Print and shaded views of the part. All mm, measured from the part's lowest x, y and z. A direction names the side the tool comes from. Give positions to 0.01 mm unless a question says otherwise; leave off trailing zeros. Write each loop counter-clockwise with the first axis right and the second up, starting at its lowest first coordinate (ties: lowest second). Pieces come first, ordered by that corner, then holes.
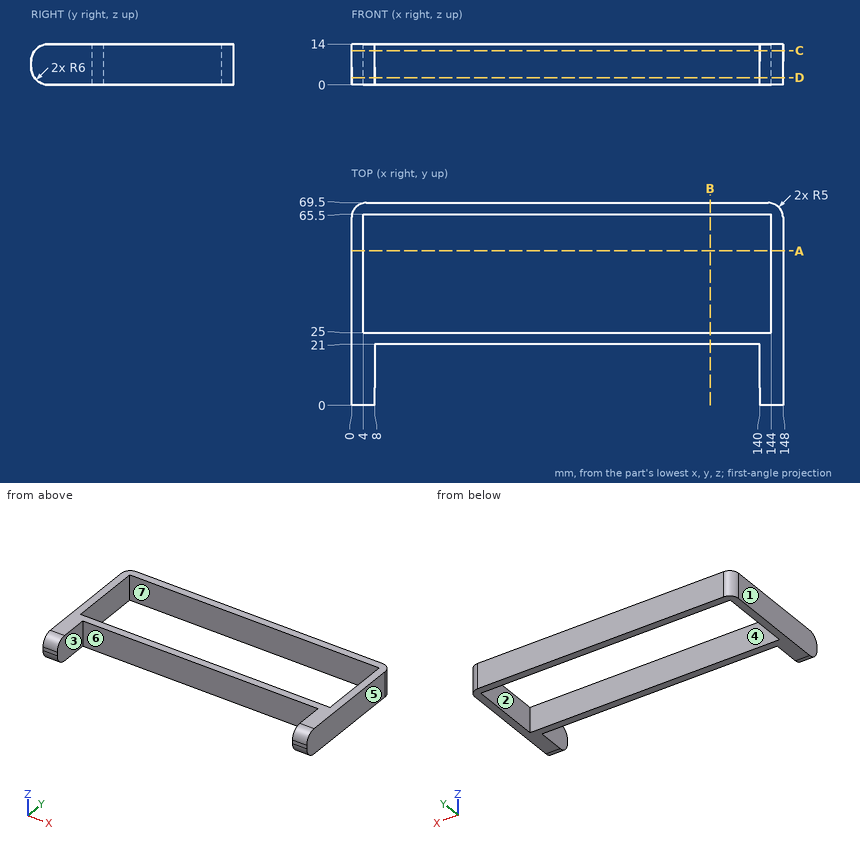
1. Saw through at C-C on z = 11.75. Give the cut face in (x, y), plus the area to 3 significant figures.
2. 3-axis set-ups, long thin cutter, end or side, ignore diameter. For the marked faces 1, 2 and 3: which of +Z, -Z, +X, -X, +Y, -Y reach the whole face in a straight line?
3. Saw through at D-D on z = 2.5. Give the cut face in (x, y), plus the area to 3 significant figures.
4. Saw through at A-A on y = 53. Give the cut face in (x, z), plus the area to 3 significant figures.
5. Drill centre lines: line 1 along Y through (x, z) = (42.5, 13); line 2 along X through (y, z) = (37, 8.75); line 3 along X through (y, z) = (15, 3.25). Where is each one in solid material? Low to high.
6. Mould opens along Y. For the marked faces 4, 5, 6 and 7 say: pulls with the +Y half, pulls with the -Y half, needs draft (parallel to the pull), parting line crosses it, or undercut.
7. Saw through at B-B on x = 123. Give the cut face in (y, z), plus the area to 3 significant figures.
8. Drop a flat-ended pin along its axis: pin 1 (3 mm diameter, centred on x = 132.5, z = 6, fed in from -Y). Give the stop position or say it passes through.
Outcome:
1. outline: (0, 1.32) - (8, 1.32) - (8, 21) - (140, 21) - (140, 1.32) - (148, 1.32) - (148, 64.5) arc R5 ccw to (143, 69.5) - (5, 69.5) arc R5 ccw to (0, 64.5) - close; hole (4, 25) - (144, 25) - (144, 65.5) - (4, 65.5) - close
1. area: 1,810 mm2
2. face 1: +Z, -Z, -X, +Y, -Y
2. face 2: +Z, -Z
2. face 3: +Z, -Z, -Y
3. outline: (0, 1.13) - (8, 1.13) - (8, 21) - (140, 21) - (140, 1.13) - (148, 1.13) - (148, 64.5) arc R5 ccw to (143, 69.5) - (5, 69.5) arc R5 ccw to (0, 64.5) - close; hole (4, 25) - (144, 25) - (144, 65.5) - (4, 65.5) - close
3. area: 1,820 mm2
4. outline: (0, 0) - (4, 0) - (4, 14) - (0, 14) - close; (144, 0) - (148, 0) - (148, 14) - (144, 14) - close
4. area: 112 mm2
5. line 1: y = 21 to 25, 65.5 to 69.5
5. line 2: x = 0 to 4, 144 to 148
5. line 3: x = 0 to 8, 140 to 148
6. face 4: undercut
6. face 5: needs draft
6. face 6: pulls with the -Y half
6. face 7: undercut
7. outline: (21, 0) - (25, 0) - (25, 14) - (21, 14) - close; (65.5, 0) - (69.5, 0) - (69.5, 14) - (65.5, 14) - close
7. area: 112 mm2
8. pin 1: stops at y = 21
